Job drawing, mm, ordinate dimensions from the low corner. One solid piece. A direction names the side the tool comes from. Coordinates: 2 decimals unless noted, no trailing zeros. Order: outer loops, then holes, each group sorted by start corner. A loop starts at its lowest first (then second) coordinate and runs counter-clockwise, first axis right, second up. Notation, with made-up numbers: (29, -8) - (81, -8) arc R14 ccw to (81, 13) - close; hole circle Ø6 at (-32, -20). An arc over 180 degrees is marked (long way). Use one line per item in the form item = value.
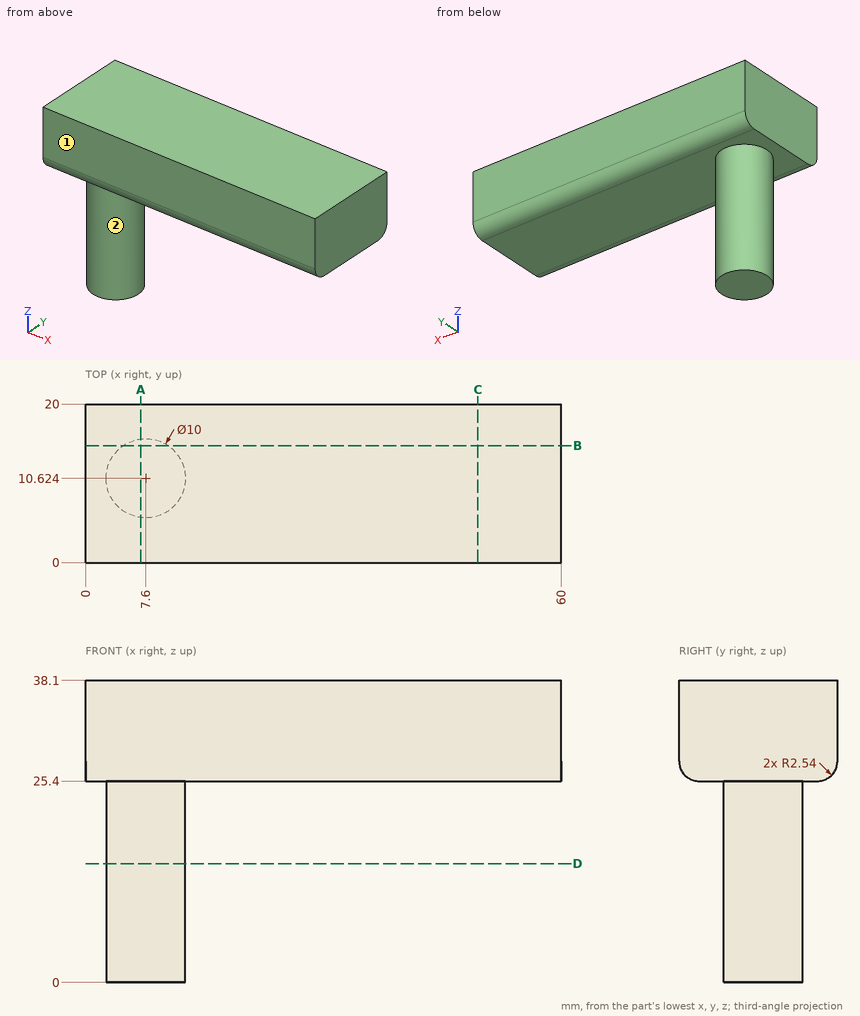
Item 1: Cut at C-C, the plane x = 49.5. Write the cut outline in (y, z), plus the area to 3 significant figures.
Derived:
outline = (0, 27.94) arc R2.54 ccw to (2.54, 25.4) - (17.46, 25.4) arc R2.54 ccw to (20, 27.94) - (20, 38.1) - (0, 38.1) - close
area = 251 mm²
Item 2: Cut at B-B, the plane y = 14.75. Write the cut outline in (x, z).
Derived:
outline = (0, 25.4) - (4.78, 25.4) - (4.78, 0) - (10.42, 0) - (10.42, 25.4) - (60, 25.4) - (60, 38.1) - (0, 38.1) - close
Item 3: Drop flat-ended pins along their axis: pin 1 (5 mm diameter, centred on x = 17, y = 8.5, fed in from -Z); pin 2 (1 mm diameter, centred on y = 5.5, z = 21, fed in from +X); pin 3 (5 mm diameter, centred on y = 7, z = 15, fed in from +X). Give the stop position or say it passes through.
Derived:
pin_1 = 25.4
pin_2 = 9.5
pin_3 = 12.47
Item 4: Cut at A-A, the plane x = 7. Write the cut outline in (y, z).
Derived:
outline = (0, 27.94) arc R2.54 ccw to (2.54, 25.4) - (5.66, 25.4) - (5.66, 0) - (15.59, 0) - (15.59, 25.4) - (17.46, 25.4) arc R2.54 ccw to (20, 27.94) - (20, 38.1) - (0, 38.1) - close
Item 5: Cut at D-D, the plane z = 15. Write the cut outline in (x, y).
Derived:
outline = circle Ø10 at (7.6, 10.62)
Item 6: 3-axis set-ups, long thin cutter, end or side, ignore diameter. For the marked faces 1 and 2: which of +Z, -Z, +X, -X, +Y, -Y reach the whole face in a straight line?
Derived:
face_1 = +Z, -Z, +X, -X, -Y
face_2 = -Z
Item 7: Drill centre lines: line 1 (Z direction, x = 46, y = 9); line 2 (Y direction, x = 9.5, z = 19.5); line 3 (X direction, y = 13.75, z = 7.5). Where is each one in solid material? Low to high. Write a range as [from, to].
Derived:
line_1 = [25.4, 38.1]
line_2 = [6, 15.25]
line_3 = [3.7, 11.5]
